from build123d import *

# Parameters (mm, degrees)
F0_W     = 27.7622
F0_H     = 23.1902
F1_DEPTH = 1.27
F2_DEPTH = 3.81
F0_W_2   = 9.1059
F0_H_2   = 38.9382
F0_R     = 1.905
F3_DEPTH = 1.27
F4_R     = 5.08


with BuildPart() as f1:
    # F0 (on Top) → F1 (new body)
    with BuildSketch(Plane.XY):
        Polygon((16.9291, -16.9291), (16.9291, 16.9291), (-16.9291, 16.9291), (-16.9291, -16.9291), (-9.525, -16.9291), (9.525, -16.9291), align=None)
        with Locations((0, 2.286)):
            Rectangle(F0_W, F0_H, mode=Mode.SUBTRACT)
    extrude(amount=F1_DEPTH)

    # F0 (on Top) → F2 (join)
    with BuildSketch(Plane.XY):
        Polygon((-16.9291, 16.9291), (16.9291, 16.9291), (16.9291, -16.9291), (9.525, -16.9291), (9.525, -19.4691), (19.4691, -19.4691), (19.4691, 19.4691), (-19.4691, 19.4691), (-19.4691, -19.4691), (-9.525, -19.4691), (-9.525, -16.9291), (-16.9291, -16.9291), align=None)
    extrude(amount=F2_DEPTH)

    # F0 (on Top) → F3 (join)
    with BuildSketch(Plane.XY):
        with Locations((-24.02205, 0)):
            Rectangle(F0_W_2, F0_H_2)
        with Locations((-24.02205, -13.1191)):
            Circle(F0_R, mode=Mode.SUBTRACT)
        with Locations((-24.02205, 0)):
            Circle(F0_R, mode=Mode.SUBTRACT)
        with Locations((-24.02205, 13.1191)):
            Circle(F0_R, mode=Mode.SUBTRACT)
        with Locations((24.02205, 0)):
            Rectangle(F0_W_2, F0_H_2)
        with Locations((24.02205, -13.1191)):
            Circle(F0_R, mode=Mode.SUBTRACT)
        with Locations((24.02205, 0)):
            Circle(F0_R, mode=Mode.SUBTRACT)
        with Locations((24.02205, 13.1191)):
            Circle(F0_R, mode=Mode.SUBTRACT)
        Polygon((-16.9291, 16.9291), (16.9291, 16.9291), (16.9291, -16.9291), (9.525, -16.9291), (9.525, -19.4691), (19.4691, -19.4691), (19.4691, 19.4691), (-19.4691, 19.4691), (-19.4691, -19.4691), (-9.525, -19.4691), (-9.525, -16.9291), (-16.9291, -16.9291), align=None)
        Polygon((16.9291, -16.9291), (16.9291, 16.9291), (-16.9291, 16.9291), (-16.9291, -16.9291), (-9.525, -16.9291), (9.525, -16.9291), align=None)
        with Locations((0, 2.286)):
            Rectangle(F0_W, F0_H, mode=Mode.SUBTRACT)
    extrude(amount=F3_DEPTH)

    # F4
    f4_edges = [f1.edges().sort_by_distance(p)[0] for p in [
        (-28.575, 19.4691, 0.635),
        (-28.575, -19.4691, 0.635),
        (28.575, 19.4691, 0.635),
        (28.575, -19.4691, 0.635),
    ]]
    fillet(f4_edges, radius=F4_R)


solid = f1.part
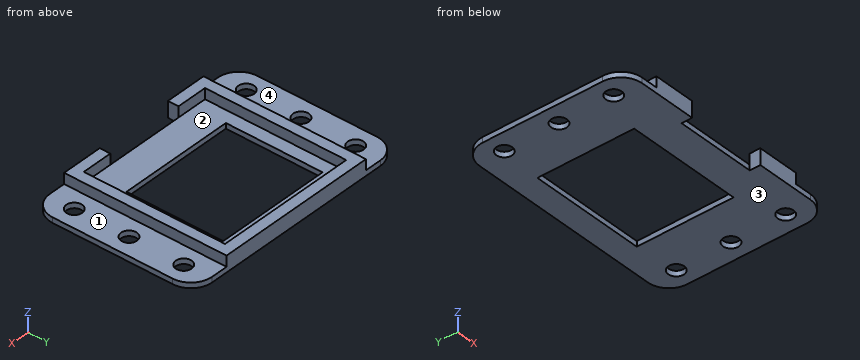
Work out the finished part from the listing and answer in its coordinate system (mm). Face numbers are marked on the shaded views. A direction names the side the tool comes from. Coordinates: 2 decimals unless noted, no trailing zeros. Loops run counter-clockwise (first coordinate to the right, second up) from the corner with the lowest first, then second, coordinate; pieces in that order, holes last. Notation, with made-up numbers: M 81.5,-34.5 L 127.5,-34.5 A22 cw 127.5,-5.5 Z; hole C 54.5,63 d11. An arc over 180 degrees is marked long. Answer in a Markdown table with one row per item. Add a question column.
1. A tool of negligible diameter and unlimited length cuts with its end or side. For the marked faces 3 and 4, from which of +Z, -Z, +X, -X, +Y, -Y can it reach the whole face along a straight path? Write none if from no direction.
2. Find section A-A, the plane y = 0. Write down the section's boundary in (x, z) (3 decimals), then the cut area to 3 significant figures.
3. Find section D-D, the plane z = 2.45. Write down the section's boundary in (x, y) (3 decimals).
4. Consider L1, parallel to Y at x = 24, z = 0.2; L2, parallel to Y at x = -11.5, z = 1.45; L3, parallel to Y at x = 9, z = 0.9. Determine where each line is inside the solid, lowest interval first.
5. Flat-ended cylindrical pins translate along their axes: P1, Ø1, axis at x = 3, z = 0.5, coming from the -Y side; P2, Ø1.3, axis at y = -3.5, z = 2.5, coming from the +X side; P3, Ø4.5, axis at x = -22, y = 2.5, coming from the +Z side. Find the tip coordinate at first contact, or state that the pin passes through.
6. The mould has two halves that part along Y. Classify the marked faces 1 and 2: pulls with the +Y half, pulls with the -Y half, needs draft (parallel to the pull), parting line crosses it, or undercut.
7. Find section C-C, the plane x = -3.5. Write down the section's boundary in (y, z).
8. Find section B-B, the plane y = -5.5. Write down the section's boundary in (x, z) (3 decimals).
Reported:
| question | item | result |
|---|---|---|
| 1 | face 3 | -Z, +X, -X, +Y, -Y |
| 1 | face 4 | +Z, -X, +Y, -Y |
| 2 | outline | M -28.575,0 L -25.927,0 L -25.927,1.27 L -28.575,1.27 Z; M -22.117,0 L -13.881,0 L -13.881,1.27 L -16.929,1.27 L -16.929,3.81 L -19.469,3.81 L -19.469,1.27 L -22.117,1.27 Z; M 13.881,0 L 22.117,0 L 22.117,1.27 L 19.469,1.27 L 19.469,3.81 L 16.929,3.81 L 16.929,1.27 L 13.881,1.27 Z; M 25.927,0 L 28.575,0 L 28.575,1.27 L 25.927,1.27 Z |
| 2 | area | 40.5 mm^2 |
| 3 | outline | M -19.469,-19.469 L -9.525,-19.469 L -9.525,-16.929 L -16.929,-16.929 L -16.929,16.929 L 16.929,16.929 L 16.929,-16.929 L 9.525,-16.929 L 9.525,-19.469 L 19.469,-19.469 L 19.469,19.469 L -19.469,19.469 Z |
| 4 | L1 | y = -19.44 to -15.02, -11.21 to -1.9, 1.9 to 11.21, 15.02 to 19.44 |
| 4 | L2 | y = -19.47 to -16.93, 16.93 to 19.47 |
| 4 | L3 | y = -16.93 to -9.31, 13.88 to 19.47 |
| 5 | P1 | stops at y = -16.93 |
| 5 | P2 | stops at x = 19.47 |
| 5 | P3 | stops at z = 1.27 |
| 6 | face 1 | needs draft |
| 6 | face 2 | undercut |
| 7 | outline | M -16.93,0 L -9.31,0 L -9.31,1.27 L -16.93,1.27 Z; M 13.88,0 L 19.47,0 L 19.47,3.81 L 16.93,3.81 L 16.93,1.27 L 13.88,1.27 Z |
| 8 | outline | M -28.575,0 L -13.881,0 L -13.881,1.27 L -16.929,1.27 L -16.929,3.81 L -19.469,3.81 L -19.469,1.27 L -28.575,1.27 Z; M 13.881,0 L 28.575,0 L 28.575,1.27 L 19.469,1.27 L 19.469,3.81 L 16.929,3.81 L 16.929,1.27 L 13.881,1.27 Z |
